```python
from build123d import *

# Parameters (mm, degrees)
BASPROSKE_W             = 10
BASPROSKE_H             = 11
TOOTHCUT_DEPTH          = 19.493242009
TEETHCUTS_COUNT         = 20
TEETHCUTS_ANGLE         = 342
BORSKE_R                = 0.4
BORE_DEPTH              = 50.0000508
CROQUIS1_R              = 2
SALIENTE_EXTRUIR1_DEPTH = 10
CROQUIS2_R              = 2
CORTAR_EXTRUIR1_DEPTH   = 10


with BuildPart() as part:
    # BasProSke → Base-Revolve (revolve)
    with BuildSketch(Plane(origin=(0, 0, 0), x_dir=(1, 0, 0), z_dir=(0, 1, 0)), mode=Mode.PRIVATE) as base_revolve_sk:
        with Locations((5, 5.5)):
            Rectangle(BASPROSKE_W, BASPROSKE_H)
    revolve(base_revolve_sk.sketch.rotate(Axis((-10, 0, 0), (1, 0, 0)), 180), axis=Axis((-10, 0, 0), (1, 0, 0)))

    # TooCutSke → ToothCut (cut, through all)
    with BuildSketch(Plane(origin=(0, 0, 0), x_dir=(0, 0, -1), z_dir=(1, 0, 0))):
        with BuildLine():
            ThreePointArc((0.499924007, 8.734705318), (0, 8.749), (-0.499924007, 8.734705318))
            ThreePointArc((-0.499924007, 8.734705318), (-0.824302243, 9.905497836), (-1.485192705, 10.924909509))
            ThreePointArc((-1.485192705, 10.924909509), (0, 11.0254), (1.485192705, 10.924909509))
            ThreePointArc((1.485192705, 10.924909509), (0.824302243, 9.905497836), (0.499924007, 8.734705318))
        make_face()
    toothcut = extrude(amount=TOOTHCUT_DEPTH, mode=Mode.SUBTRACT)

    # TeethCuts: ToothCut ×20 about axis
    teethcuts_axis = Axis((-10, 0, 0), (1, 0, 0))
    for i in range(1, TEETHCUTS_COUNT):
        add(toothcut.rotate(teethcuts_axis, i * TEETHCUTS_ANGLE / (TEETHCUTS_COUNT - 1)), mode=Mode.SUBTRACT)

    # BorSke → Bore (cut, symmetric)
    with BuildSketch(Plane(origin=(0, 0, 0), x_dir=(0, 0, -1), z_dir=(1, 0, 0))):
        with Locations(Location((0, 0, 0), (0, 0, 180))):
            Circle(BORSKE_R)
    extrude(amount=BORE_DEPTH, both=True, mode=Mode.SUBTRACT)

    # Croquis1 → Saliente-Extruir1 (add)
    with BuildSketch(Plane(origin=(10, 0, 0), x_dir=(0, 0, -1), z_dir=(1, 0, 0))):
        with BuildLine():
            Line((38.725361299, 11.195820305), (-0.782172325, 4.938441703))
            ThreePointArc((-0.782172325, 4.938441703), (-4.938441703, -0.782172325), (0.782172325, -4.938441703))
            Line((0.782172325, -4.938441703), (40.289705949, 1.318936899))
            ThreePointArc((40.289705949, 1.318936899), (44.445975327, 7.039550927), (38.725361299, 11.195820305))
        make_face()
        Circle(CROQUIS1_R, mode=Mode.SUBTRACT)
        with Locations((39.507533624, 6.257378602)):
            Circle(CROQUIS1_R, mode=Mode.SUBTRACT)
    extrude(amount=-SALIENTE_EXTRUIR1_DEPTH)

    # Croquis2 → Cortar-Extruir1 (cut)
    with BuildSketch(Plane(origin=(10, 0, 0), x_dir=(0, 0, -1), z_dir=(1, 0, 0))):
        Circle(CROQUIS2_R)
    extrude(amount=-CORTAR_EXTRUIR1_DEPTH, mode=Mode.SUBTRACT)


solid = part.part
```
Build history of the part. All positions in model axes, mm. A direction names the side the tool comes from. Round coordinates to 2 decimals unless told otherwise and drop trailing zeros. Write each loop counter-clockwise with the first axis right and the second up, starting at its lowest first coordinate (ties: lowest second). Pieces come first, ordered by that corner, then holes. Notation, with made-up numbers: (44.5, -22.5) - (97.5, -22.5) arc R21 ccw to (97.5, 3.5) - close; hole circle Ø10 at (38.5, 84). An arc over 180 degrees is marked (long way). Write each question's results on one line, items separated by ' | '. Start each with the question number.
Item 1: Which spindle directions (+Z, -Z, +X, -X, +Y, -Y) get a long thin tool onto all of the face, cutting with end or side? Do faces 1 (the face through (4.93, 7.53, -6.49)), 2 (the face through (4.93, 9.677, 2.277)), 3 (the face through (0, 3, -10)), 4 (the face through (4.93, -9.14, -3.82)), 5 (the face through (4.93, -6.461, 7.513)). Say none if no direction does.
Item 2: Saw through at A-A (z = 0). Write the cut outline in (x, y), and give its area (3 significant figures).
Item 3: Saw through at B-B (x = 3.5). State how many separate pieces and enclosed holes the cut face has, and give its area (3 significant figures).
Item 4: Wall check: L1, parallel to Z at x = 7.75, y = -7; L2, parallel to Y at x = 2.5, z = 0; L3, parallel to Z at x = 6, y = -9.75. Give the ranges that are in metal, low to high. Write a range as [from, to].
Item 5: Saw through at C-C (z = -26). Write the cut outline in (x, y), and give its area (3 significant figures).
Item 6: Drop flat-ended pins along their axis: P1, Ø3, axis at x = 1.5, y = -4, coming from the +Z side; P2, Ø4, axis at x = 8, z = -1, coming from the +Y side; P3, Ø4.5, axis at y = 6.26, z = -39.51, coming from the +X side. Give the stop position or say it passes through.
Item 7: Mould opens along Z. For faces 6 (the face through (4.93, -8.47, 5.15)), 7 (the face through (10, 3, -10)), 8 (the face through (4.93, 0.01, 8.75)) say: pulls with the +Z half, pulls with the -Z half, needs draft (parallel to the pull), parting line crosses it, or undercut.
Results are:
1) face 1: +X, -X, +Y | face 2: +X, -X | face 3: +Z, -Z, -X, +Y, -Y | face 4: +X, -X, -Y | face 5: +Z, +X, -X
2) outline: (0, -8.75) - (10, -8.75) - (10, -2) - (0, -2) - close; (0, 2) - (10, 2) - (10, 8.75) - (0, 8.75) - close | area: 135 mm²
3) separate pieces: 1 | enclosed holes: 2 | area: 624 mm²
4) L1: z = [-7.78, -5.77], [-5.25, 5.25], [5.77, 7.78] | L2: y = [-8.75, -2], [2, 8.75] | L3: z = [-5.09, -4.51], [-2.27, -0.76], [0.76, 2.27], [4.51, 5.09]
5) outline: (0, -0.94) - (10, -0.94) - (10, 9.18) - (0, 9.18) - close | area: 101 mm²
6) P1: stops at z = 9.92 | P2: stops at y = 10.9 | P3: stops at x = 10
7) face 6: undercut | face 7: needs draft | face 8: pulls with the +Z half
